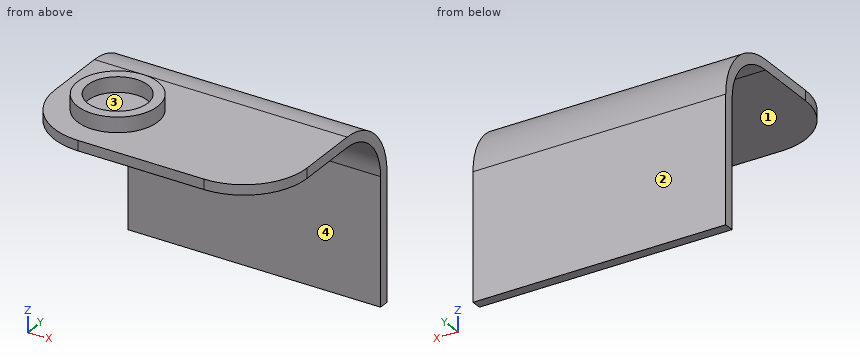
from build123d import *

# Parameters (mm, degrees)
F0_W     = 50
F0_H     = 25
F1_DEPTH = 2
F3_DEPTH = 50
F4_R     = 12.5
F5_R     = 7.95
F5_R_2   = 5.95
F6_DEPTH = 3


with BuildPart() as f1:
    # F0 (on Front) → F1 (new body)
    with BuildSketch(Plane.XZ):
        with Locations((-25, 12.5)):
            Rectangle(F0_W, F0_H)
    extrude(amount=F1_DEPTH)

    # F2 (on Right) → F3 (join, through all)
    with BuildSketch(Plane.YZ):
        with BuildLine():
            Line((-2, 25), (0, 25))
            ThreePointArc((0, 25), (-3.6611652352, 33.8388347648), (-12.5, 37.5))
            Line((-12.5, 37.5), (-37.5, 37.5))
            Line((-37.5, 37.5), (-37.5, 35.5))
            Line((-37.5, 35.5), (-12.5, 35.5))
            ThreePointArc((-12.5, 35.5), (-5.0753787975, 32.4246212025), (-2, 25))
        make_face()
    extrude(amount=-F3_DEPTH)

    # F4
    f4_edges = [f1.edges().sort_by_distance(p)[0] for p in [
        (-50, -37.5, 36.5),
        (0, -37.5, 36.5),
    ]]
    fillet(f4_edges, radius=F4_R)

    # F5 (on face) → F6 (join)
    with BuildSketch(Plane.XY.offset(37.5)):
        with Locations((-37.5, -25)):
            Circle(F5_R)
        with Locations((-37.5, -25)):
            Circle(F5_R_2, mode=Mode.SUBTRACT)
    extrude(amount=F6_DEPTH)


solid = f1.part
Read the model definition and answer for the solid it produces. Units are mm, in the model's axes. Face numbers are marked on the shaded views. A direction names the side the tool comes from. Coordinates: 2 decimals unless noted, no trailing zeros. Order: outer loops, then holes, each group sorted by start corner. A loop starts at its lowest first (then second) coordinate and runs counter-clockwise, first axis right, second up. Notation, with made-up numbers: M 22.25,25.5 L 55.25,25.5 A9 cw 55.25,32.5 Z; hole C 49,42 d10. An arc over 180 degrees is marked long. Put each result on its own line as item: value. Start each with the question number.
Item 1: Section B-B, the plane y = -29.5 is taken. Determine the outline of the cut face in (x, z).
Item 2: Section A-A, the plane x = -25.5 is taken. Determine the outline of the cut face in (y, z).
Item 3: Section C-C, the plane z = 15 is taken. Determine the outline of the cut face in (x, y).
Item 4: Consider probe 1 along Y at (x, z) = (-37.5, 39.15); probe 2 along Y at (x, z) = (-19.5, 9.5); probe 3 along Z at (x, y) = (-28.5, -31.5). Determine where each line is inside the solid, lowest interval first. Write a range as [from, to].
Item 5: Given pin 1 Ø3 at (x, y) = (-35, -12.5) entering from -Z; pin 2 Ø2 at (x, y) = (-44.5, -19) entering from -Z; pin 3 Ø6 at (x, y) = (-37, -23.5) entering from +Z, each flat-ended and moving along its own axis, determine where each tip first touches the part or whether it passes through.
Item 6: For the marked faces 1 and 2, determine the directions among +Z, -Z, +X, -X, +Y, -Y from which every point of the face is accessible in a straight line to the end or side of a thin tool.
Item 7: Section D-D, the plane x = -8 is taken. Determine the outline of the cut face in (y, z), plus the area to 3 significant figures.
Item 8: The mould has two halves that part along X. Classify the marked faces 3 and 4: +X half, -X half, draft (parallel to the pull), parting line (faces both ways), or undercut.
Computed:
1. outline: M -49.16,35.5 L -0.84,35.5 L -0.84,37.5 L -30.95,37.5 L -30.95,40.5 L -33.61,40.5 L -33.61,37.5 L -41.39,37.5 L -41.39,40.5 L -44.05,40.5 L -44.05,37.5 L -49.16,37.5 Z
2. outline: M -37.5,35.5 L -12.5,35.5 A10.5 cw -2,25 L -2,0 L 0,0 L 0,25 A12.5 ccw -12.5,37.5 L -37.5,37.5 Z
3. outline: M -50,-2 L 0,-2 L 0,0 L -50,0 Z
4. probe 1: y = [-32.95, -30.95], [-19.05, -17.05]
4. probe 2: y = [-2, 0]
4. probe 3: z = [35.5, 37.5]
5. pin 1: stops at z = 35.39
5. pin 2: stops at z = 35.5
5. pin 3: stops at z = 37.5
6. face 1: -Z, +X, -X, -Y
6. face 2: +Z, -Z, +X, -X, +Y
7. outline: M -36.66,35.5 L -12.5,35.5 A10.5 cw -2,25 L -2,0 L 0,0 L 0,25 A12.5 ccw -12.5,37.5 L -36.66,37.5 Z
7. area: 134 mm2
8. face 3: undercut
8. face 4: draft
